Here's how the part is built. I have some questions about the finished solid (model axes, mm). Face numbers are marked on the shaded views. A direction names the side the tool comes from. Coordinates: 2 decimals unless noted, no trailing zeros. Loops run counter-clockwise (first coordinate to the right, second up) from the corner with the lowest first, then second, coordinate; pieces in that order, holes last. Notation, with made-up numbers: (2, -35) -> (39, -35) arc R21 cw to (39, -5) -> close; hole circle Ø2 at (45, -18). An arc over 180 degrees is marked (long way). Use CSV: the item, a comma, the result in double quotes. Start each with the question number.
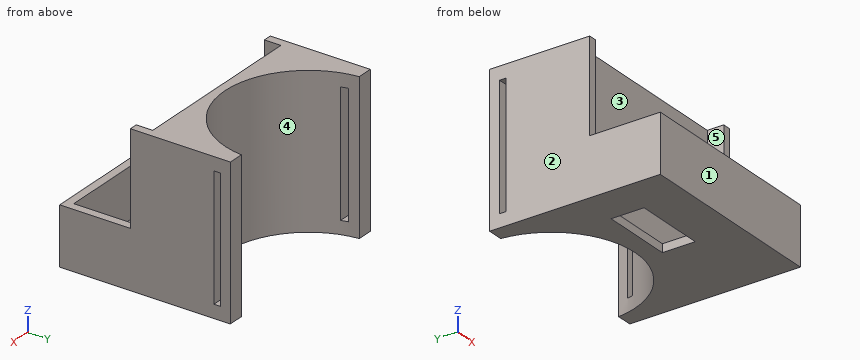
from build123d import *

# Parameters (mm, degrees)
F0_W      = 55
F0_H      = 55
F1_DEPTH  = 24
F2_W      = 60
F2_H      = 29
F3_DEPTH  = 2.5
F4_DEPTH  = 15
F5_W      = 22
F5_H      = 10
F6_DEPTH  = 2.5
F7_W      = 2.5
F7_H      = 5
F8_DEPTH  = 28
F9_DEPTH  = 25.4
F11_DEPTH = 46
F12_W     = 2
F12_H     = 37.5
F13_DEPTH = 60
F14_DEPTH = 24


with BuildPart() as f1:
    # F0 (on Front) → F1 (new body)
    with BuildSketch(Plane.XZ):
        Rectangle(F0_W, F0_H)
    extrude(amount=F1_DEPTH)

    # F2 (on face) → F3 (join)
    with BuildSketch(Plane(origin=(0, 0, -27.5), x_dir=(1, 0, 0), z_dir=(0, 0, -1))):
        with Locations((0, 12)):
            Rectangle(F2_W, F2_H)
    extrude(amount=F3_DEPTH)

    # F2 (on face) → F4 (join)
    with BuildSketch(Plane(origin=(0, 0, -27.5), x_dir=(1, 0, 0), z_dir=(0, 0, -1))):
        with Locations((0, 12)):
            Rectangle(F2_W, F2_H)
    extrude(amount=-F4_DEPTH)

    # F5 (on face) → F6 (cut)
    with BuildSketch(Plane(origin=(0, 0, -30), x_dir=(1, 0, 0), z_dir=(0, 0, -1))):
        with Locations((-7, 8)):
            Rectangle(F5_W, F5_H)
    extrude(amount=-F6_DEPTH, mode=Mode.SUBTRACT)

    # F7 (on face) → F8 (join)
    with BuildSketch(Plane.XY.offset(-12.5)):
        Polygon((30, 2.5), (-30, 2.5), (-30, 0), (-27.5, 0), (27.5, 0), (30, 0), align=None)
        with Locations((-28.75, -2.5)):
            Rectangle(F7_W, F7_H)
        with Locations((28.75, -2.5)):
            Rectangle(F7_W, F7_H)
    extrude(amount=F8_DEPTH)

    # F9 (add): a face of the model
    f9_faces = [f1.faces().sort_by_distance(p)[0] for p in [
        (0, 2.5, -7.25),
    ]]
    extrude(f9_faces, amount=F9_DEPTH)

    # F10 (on face) → F11 (cut)
    with BuildSketch(Plane.XY.offset(15.5)):
        with BuildLine():
            Line((-25.4, 27.9), (25.4, 27.9))
            ThreePointArc((25.4, 27.9), (0, 53.3), (-25.4, 27.9))
        make_face()
        with BuildLine():
            Line((30, 27.9), (25.4, 27.9))
            ThreePointArc((25.4, 27.9), (25.3691485346, 26.6484798728), (25.2766690844, 25.4))
            Line((25.2766690844, 25.4), (30, 25.4))
            Line((30, 25.4), (30, 27.9))
        make_face()
        with BuildLine():
            ThreePointArc((25.2766690844, 25.4), (25.3691485346, 26.6484798728), (25.4, 27.9))
            Line((25.4, 27.9), (-25.4, 27.9))
            ThreePointArc((-25.4, 27.9), (-25.3691485346, 26.6484798728), (-25.2766690844, 25.4))
            Line((-25.2766690844, 25.4), (25.2766690844, 25.4))
        make_face()
        with BuildLine():
            ThreePointArc((-25.2766690844, 25.4), (-25.3691485346, 26.6484798728), (-25.4, 27.9))
            Line((-25.4, 27.9), (-30, 27.9))
            Line((-30, 27.9), (-30, 25.4))
            Line((-30, 25.4), (-25.2766690844, 25.4))
        make_face()
        with BuildLine():
            ThreePointArc((-25.2766690844, 25.4), (0, 2.5), (25.2766690844, 25.4))
            Line((25.2766690844, 25.4), (-25.2766690844, 25.4))
        make_face()
    extrude(amount=-F11_DEPTH, mode=Mode.SUBTRACT)

    # F12 (on face) → F13 (cut)
    with BuildSketch(Plane.YZ.offset(30)):
        with Locations((21.4, -7.25)):
            Rectangle(F12_W, F12_H)
    extrude(amount=-F13_DEPTH, mode=Mode.SUBTRACT)

    # F0 (on Front) → F14 (cut)
    with BuildSketch(Plane.XZ):
        Rectangle(F0_W, F0_H)
    extrude(amount=F14_DEPTH, mode=Mode.SUBTRACT)


solid = f1.part
1) Please list where these lines run through material, in increasing order: L1, parallel to X at y = -5.5, z = -26; L2, parallel to Y at x = 19.5, z = -18.5; L3, parallel to Y at x = 0, z = 1.5. Write a range as [from, to].
2) Which directions (+Z, -Z, +X, -X, +Y, -Y) give clear straight access to the entire face, cutting with the end or side of a thin tool? Please do the marked faces 4 and 5.
3) I want a section at D-D, the plane x = -10. Please give me the cut outline in (y, z), plus the area to 3 significant figures.
4) I want a section at C-C, the plane z = -2.5. Please give me the cut outline in (x, y).
5) I want a section at B-B, the plane z = -21.5. Please give me the cut outline in (x, y).
6) For P1, Ø12, axis at x = -11, z = -23, coming from the +Y side; P2, Ø12, axis at x = 7.5, z = -3.5, coming from the -Y side; P3, Ø1.2, axis at x = -3.5, z = -28.5, coming from the +Y side, each with a flat end and sliding along its axis, tell me the tip position at first contact or that it passes through.
7) Thinking about a two-plate mould opening in Y: for the marked faces 1, 2 and 3, which applies, pulls with the +Y half, pulls with the -Y half, needs draft (parallel to the pull), parting line crosses it, or undercut?
8) I want a section at A-A, the plane y = -11.5. Please give me the cut outline in (x, z), plus the area to 3 significant figures.
Return value:
1,L1,"x = [-30, -27.5], [27.5, 30]"
1,L2,"y = [-26.5, -24], [0, 11.62]"
1,L3,"y = [0, 2.5]"
2,face 4,"+Z, -Z, +Y"
2,face 5,"+Z"
3,outline,"(-26.5, -30) -> (-13, -30) -> (-13, -27.5) -> (-24, -27.5) -> (-24, -12.5) -> (-26.5, -12.5) -> close; (-3, -30) -> (4.55, -30) -> (4.55, 15.5) -> (0, 15.5) -> (0, -27.5) -> (-3, -27.5) -> close"
3,area,"286 mm²"
4,outline,"(-30, -5) -> (-27.5, -5) -> (-27.5, 0) -> (27.5, 0) -> (27.5, -5) -> (30, -5) -> (30, 20.4) -> (24.27, 20.4) arc R25.4 cw to (-24.27, 20.4) -> (-30, 20.4) -> close; (-30, 22.4) -> (-24.8, 22.4) arc R25.4 cw to (-25.28, 25.4) -> (-30, 25.4) -> close; (24.8, 22.4) -> (30, 22.4) -> (30, 25.4) -> (25.28, 25.4) arc R25.4 cw to start"
5,outline,"(-30, -26.5) -> (30, -26.5) -> (30, 20.4) -> (24.27, 20.4) arc R25.4 cw to (-24.27, 20.4) -> (-30, 20.4) -> close; (-30, 22.4) -> (-24.8, 22.4) arc R25.4 cw to (-25.28, 25.4) -> (-30, 25.4) -> close; (24.8, 22.4) -> (30, 22.4) -> (30, 25.4) -> (25.28, 25.4) arc R25.4 cw to start; hole (-27.5, -24) -> (27.5, -24) -> (27.5, 0) -> (-27.5, 0) -> close"
6,P1,"stops at y = 9.03"
6,P2,"stops at y = 0"
6,P3,"stops at y = 2.83"
7,face 1,"pulls with the -Y half"
7,face 2,"needs draft"
7,face 3,"undercut"
8,outline,"(-30, -30) -> (-18, -30) -> (-18, -27.5) -> (-27.5, -27.5) -> (-27.5, -12.5) -> (-30, -12.5) -> close; (4, -30) -> (30, -30) -> (30, -12.5) -> (27.5, -12.5) -> (27.5, -27.5) -> (4, -27.5) -> close"
8,area,"170 mm²"
